Verification items for this drawing (mm, ordinates from the low corner). Round coordinates to 2 decimals unless told otherwise and drop trailing zeros. Write each loop counter-clockwise with the first axis right and the second up, starting at its lowest first coordinate (ties: lowest second). Pieces come first, ordered by that corner, then holes.
Item 1: Cross-section at D-D (x = 3). Enter the section's corners in (y, z) (1 decimal).
Item 2: Scan lines: probe 1 along Y at (x, z) = (21.25, 13); probe 2 along Z at (x, y) = (18.75, 7.75) (1 decimal); probe 3 along Z at (x, y) = (15.75, 6.5). Record each from-to range of solid material in increasing order.
Item 3: Cross-section at C-C (z = 7.5). Enter the section's corners in (x, y) (1 decimal).
Item 4: Draft check along X on the marked faces 1, 2 and 3. Enter one of: pulls with the +X half, pulls with the -X half, needs draft (parallel to the pull), parting line crosses it, or undercut.
Item 5: Cross-section at B-B (x = 10.25). Enter the section's corners in (y, z) (1 decimal).
Item 6: Cross-section at A-A (z = 15). Enter the section's corners in (x, y) (1 decimal).
Item 7: Depth check by flat-ended pin: P1, Ø4, axis at x = 5.5, y = 7.5, coming from the -Z side; P2, Ø7, axis at x = 16.5, z = 13, coming from the +Y side; P3, Ø1.5, axis at y = 6.5, z = 18, coming from the +X side (1 decimal); P4, Ø4, axis at x = 5, z = 17, coming from the -Y side. Enter the tip coordinate at first touch or a pass-through.
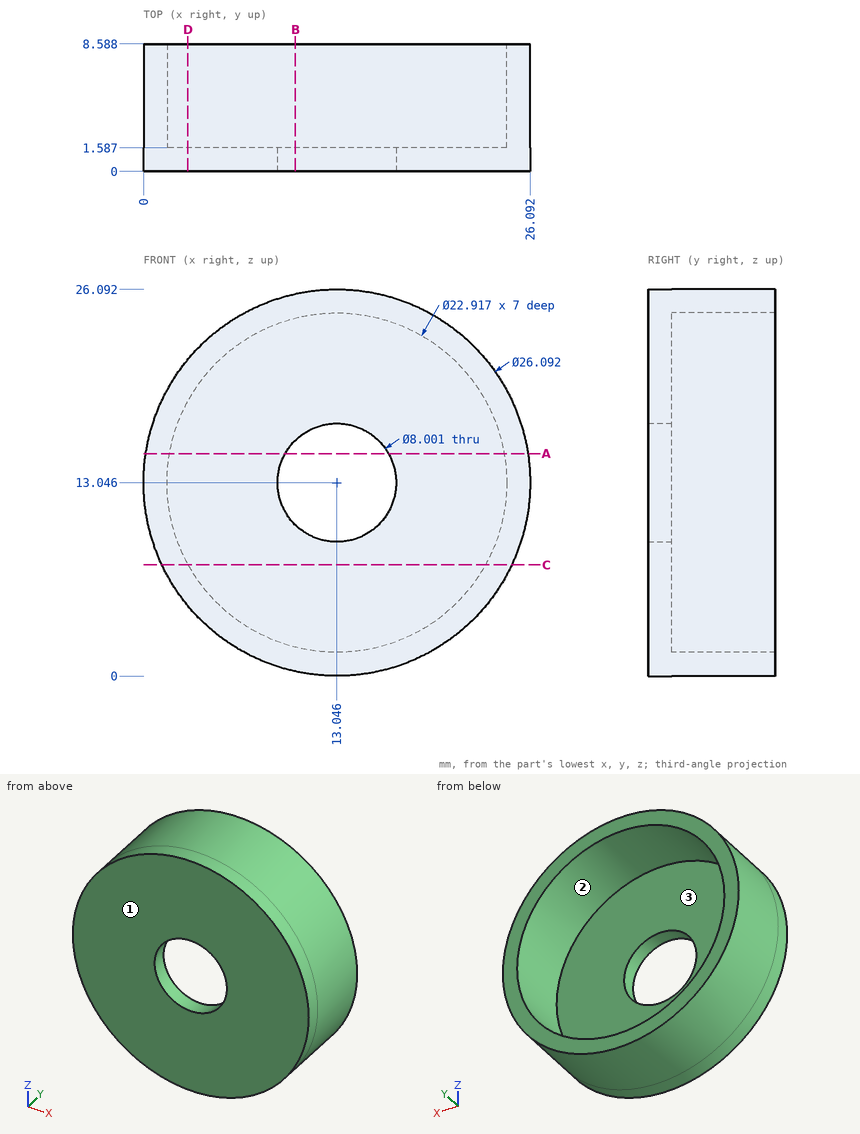
Resolved:
1. outline: (0, 4.7) - (8.6, 4.7) - (8.6, 7.5) - (1.6, 7.5) - (1.6, 18.6) - (8.6, 18.6) - (8.6, 21.4) - (0, 21.4) - close
2. probe 1: y = 0 to 1.59
2. probe 2: z = 1.3 to 3.1, 23 to 24.8
2. probe 3: z = 0.28 to 1.91, 24.18 to 25.81
3. outline: (1.2, 0) - (24.9, 0) - (24.9, 8.6) - (23.1, 8.6) - (23.1, 1.6) - (3, 1.6) - (3, 8.6) - (1.2, 8.6) - close
4. face 1: needs draft
4. face 2: undercut
4. face 3: undercut
5. outline: (0, 0.3) - (8.6, 0.3) - (8.6, 1.9) - (1.6, 1.9) - (1.6, 10.2) - (0, 10.2) - close; (0, 15.9) - (1.6, 15.9) - (1.6, 24.2) - (8.6, 24.2) - (8.6, 25.8) - (0, 25.8) - close
6. outline: (0.1, 0) - (9.6, 0) - (9.6, 1.6) - (1.8, 1.6) - (1.8, 8.6) - (0.1, 8.6) - close; (16.5, 0) - (25.9, 0) - (25.9, 8.6) - (24.3, 8.6) - (24.3, 1.6) - (16.5, 1.6) - close
7. P1: stops at z = 1.24
7. P2: stops at y = 1.59
7. P3: stops at x = 25.4
7. P4: stops at y = 0
